Autodesk Inventor part; units mm, degrees
ref_plane "YZ Plane" through (0, 0, 0) normal (1, 0, 0) x (0, 1, 0)
ref_plane "XZ Plane" through (0, 0, 0) normal (0, 1, 0) x (-1, 0, 0)
ref_plane "XY Plane" through (0, 0, 0) normal (0, 0, 1) x (1, 0, 0)
sketch "Sketch1" plane through (0, 0, 0) normal (0, 0, 1) x (1, 0, 0)
  line L0 (0, 0) -> (0, 50.8)
  line L1 (0, 50.8) -> (4.7625, 50.8)
  line L2 (4.7625, 50.8) -> (4.7625, 4.7625)
  line L3 (4.7625, 4.7625) -> (19.05, 4.7625)
  line L4 (19.05, 4.7625) -> (19.05, 0)
  line L5 (19.05, 0) -> (0, 0)
  dimension "d0" = 4.7625
  dimension "d1" = 19.05
  dimension "d2" = 50.8
  dimension "d3" = 4.7625
extrude "Extrusion1" add sketch "Sketch1" along normal blind 76.2
sketch "Sketch2" plane through (4.7625, 4.7625, 0) normal (1, 0, 0) x (0, 0, -1)
  circle A0 centre (-57.15, 23.0187) radius 3.2512
  circle A1 centre (-19.05, 23.0187) radius 3.2512
  line L0 (-76.2, 0) -> (-76.2, 46.0375)
  line L1 (0, 0) -> (0, 46.0375)
  line L2 (-60.4012, 23.0187) -> (-60.4012, 29.3687)
  line L3 (-60.4012, 29.3687) -> (-64.8676, 46.0375)
  line L4 (0, 46.0375) -> (-76.2, 46.0375)
  line L5 (-53.8988, 23.0187) -> (-53.8988, 29.3687)
  line L6 (-53.8988, 29.3687) -> (-49.4324, 46.0375)
  line L7 (-22.3012, 23.0187) -> (-22.3012, 29.3687)
  line L8 (-22.3012, 29.3687) -> (-26.7676, 46.0375)
  line L9 (-11.3324, 46.0375) -> (-15.7988, 29.3687)
  line L10 (-15.7988, 29.3687) -> (-15.7988, 23.0187)
  point P0 (0, -4.7625)
  point P1 (-76.2, 23.0187)
  point P2 (0, 23.0187)
  point P3 (-76.2, 23.0187)
  dimension "d6" = 6.5024
  dimension "d7" = 6.5024
  dimension "d8" = 19.05
  dimension "d9" = 38.1
  dimension "d10" = 19.05
  dimension "d11" = 6.35
  dimension "d12" = 165
extrude "Extrusion2" cut sketch "Sketch2" against normal blind 76.2
sketch "Sketch3" plane through (4.7625, 4.7625, 0) normal (1, 0, 0) x (0, 0, -1)
  arc A0 (-22.3012, 23.0187) -> (-15.7988, 23.0187) centre (-19.05, 23.0187) ccw
  circle A1 centre (-19.05, 23.0187) radius 6.35
  arc A2 (-60.4012, 23.0187) -> (-53.8988, 23.0187) centre (-57.15, 23.0187) ccw
  circle A3 centre (-57.15, 23.0187) radius 6.35
  point P0 (0, -4.7625)
  dimension "d15" = 12.7
  dimension "d16" = 12.7
extrude "Extrusion3" cut sketch "Sketch3" against normal blind 2.3813
fillet "Fillet1" radius 3.175 4 edges at (2.3813, 50.8, 64.8676) (2.3813, 50.8, 49.4324) (2.3813, 50.8, 26.7676) (2.3813, 50.8, 11.3324)
sketch "Sketch4" plane through (4.7625, 4.7625, 0) normal (0, 1, 0) x (1, 0, 0)
  circle A0 centre (7.9375, -63.5) radius 2.4892
  line L0 (14.2875, -76.2) -> (0, -76.2)
  line L1 (14.2875, 0) -> (14.2875, -76.2)
  circle A1 centre (7.9375, -50.8) radius 2.4892
  circle A2 centre (7.9375, -38.1) radius 2.4892
  circle A3 centre (7.9375, -25.4) radius 2.4892
  circle A4 centre (7.9375, -12.7) radius 2.4892
  circle A5 centre (7.9375, 0) radius 2.4892 construction
  line L2 (-4.7625, -67.3038) -> (-4.7625, -76.2)
  line L3 (-4.7625, -67.3038) -> (-4.7625, -64.237)
  line L4 (-4.7625, -60.4012) -> (-4.7625, -53.8988)
  line L5 (0, -64.237) -> (-4.7625, -64.237)
  line L6 (0, -60.4012) -> (0, -64.237)
  line L7 (0, -60.4012) -> (-4.7625, -60.4012)
  line L8 (-4.7625, -64.237) -> (-4.7625, -60.4012)
  point P0 (-4.7625, 0)
  point P1 (7.1437, -76.2)
  dimension "d20" = 4.9784
  dimension "d21" = 12.7
  dimension "d24" = 12.7
  dimension "d33" = 12.7
extrude "Extrusion4" cut sketch "Sketch4" against normal through all contours A0 | A1 | A2 | A3 | A4
fillet "Fillet2" radius 6.35 4 edges at (19.05, 2.3813, 76.2) (19.05, 2.3813, 0) (2.3813, 50.8, 76.2) (2.3813, 50.8, 0)
equation "\"d8\" = d10"
properties part number "BUMP_006_Bigbracket" material "Aluminum 6061"
Geometry check sheet. Reference: the model listing, model coordinates, mm. A direction names the side the tool comes from. Round coordinates to 2 decimals unless told otherwise and drop trailing zeros. Loops run counter-clockwise (first coordinate to the right, second up) from the corner with the lowest first, then second, coordinate; pieces in that order, holes last. Notation, with made-up numbers: (-30.75, -6.75) - (17.25, -6.75) arc R11 ccw to (17.25, 13.25) - close; hole circle Ø5 at (-21.75, -20.5). An arc over 180 degrees is marked (long way). Write each question's results on one line, items separated by ' | '. Start each with the question number.
Q1. Thickness scan on line 1 (Z direction, x = 12.7, y = 2.3); line 2 (X direction, y = 3, z = 38); line 3 (Y direction, x = 11, z = 47.5). Record the ranges inside material, lowest first. Write a range as [from, to].
Q2. Cross-section at D-D on x = 7.25. Enter the section's corners in (y, z), and give its area (3 significant figures).
Q3. Cross-section at B-B on z = 24. Enter the section's corners in (x, y).
Q4. Release check for a two-part mould opening along Y. For faces 1 (the cylindrical face through (2.41, 48.89, 1.81)), 2 (the flat face through (4.762, 28, 38)), 3 (the cylindrical face through (3.589, 21.435, 19.281)), 4 (the cylindrical face through (3.589, 21.435, 57.381)) record: +Y half, -Y half, draft (parallel to the pull), parting line (faces both ways), or undercut.
Q5. Access from +Z, -Z, +X, -X, +Y, -Y to the whole of each face (thin tool, end or side, straight path). Record for faces 5 (the cylindrical face through (2.35, 50.13, 10.85)), 6 (the flat face through (3, 18, 0)), 7 (the flat face through (2.381, 23, 19)).
Q6. Cross-section at A-A on y = 30.5. Enter the section's corners in (x, z).
Q7. Gauge pin test, flat ends, axial feed: P1, Ø4.5, axis at x = 12.7, z = 63.5, coming from the +Y side; P2, Ø6, axis at x = 14.5, z = 68, coming from the +Y side; P3, Ø9.5, axis at y = 30, z = 55.5, coming from the +X side; P4, Ø1, axis at y = 23, z = 56.5, coming from the +X side. Record the tip position at first contact, or that the pin passes through.
Q8. Cross-section at C-C on y = 38.5. Enter the section's corners in (x, z), and give its area (3 significant figures).
Answers below:
1) line 1: z = [0, 10.21], [15.19, 22.91], [27.89, 35.61], [40.59, 48.31], [53.29, 61.01], [65.99, 76.2] | line 2: x = [0, 10.21], [15.19, 19.05] | line 3: y = [0, 4.76]
2) outline: (0, 0) - (4.76, 0) - (4.76, 76.2) - (0, 76.2) - close | area: 363 mm²
3) outline: (0, 0) - (10.64, 0) - (10.64, 4.76) - (4.76, 4.76) - (4.76, 23.8) - (2.38, 23.8) - (2.38, 31.76) - (4.76, 31.76) - (4.76, 40.47) - (0, 40.47) - close; (14.76, 0) - (19.05, 0) - (19.05, 4.76) - (14.76, 4.76) - close
4) face 1: +Y half | face 2: draft | face 3: undercut | face 4: undercut
5) face 5: +X, -X, +Y | face 6: -Z, +X, -X, +Y, -Y | face 7: +X
6) outline: (0, 0) - (4.76, 0) - (4.76, 13.31) - (2.38, 13.31) - (2.38, 15.8) - (0, 15.8) - close; (0, 22.3) - (2.38, 22.3) - (2.38, 24.79) - (4.76, 24.79) - (4.76, 51.41) - (2.38, 51.41) - (2.38, 53.9) - (0, 53.9) - close; (0, 60.4) - (2.38, 60.4) - (2.38, 62.89) - (4.76, 62.89) - (4.76, 76.2) - (0, 76.2) - close
7) P1: passes through | P2: stops at y = 4.76 | P3: stops at x = 4.76 | P4: stops at x = 2.38
8) outline: (0, 0) - (4.76, 0) - (4.76, 14.63) - (0, 14.63) - close; (0, 23.47) - (4.76, 23.47) - (4.76, 52.73) - (0, 52.73) - close; (0, 61.57) - (4.76, 61.57) - (4.76, 76.2) - (0, 76.2) - close | area: 279 mm²
